Input: part model. Units: mm. Frame: model coordinates. Face numbers are marked on the shaded views. Coordinates: 2 decimals unless noted, no trailing zeros. Loops run counter-clockwise (first coordinate to the right, second up) from the corner with the lowest first, then second, coordinate; pieces in that order, holes last. Notation, with made-up numbers: (18.5, -21) - (62.5, -21) arc R24 ccw to (62.5, 3) - close; hole circle Ø11 at (79, 52.5). An arc over 180 degrees is marked (long way). Use a Markdown table: item, result. Add a question column.
1. Contact query for flat-ended pins moving along their axis: P1, Ø7.5, axis at x = 50.5, z = 7.5, coming from the -Y side; P2, Ø4, axis at x = -50.8, z = 6.35, coming from the +Y side; P3, Ø3, axis at x = 50.8, z = 6.35, coming from the -Y side (3 decimals); P4, Ø12, axis at x = -22.5, y = -18, coming from the -Z side. Output: stop coordinate, or through.
2. Section query B-B on z = 2. Return the cut outline in (x, y), then the cut area to 3 significant figures.
3. Section query C-C on x = 14.5. Return the cut outline in (y, z), then the cut area to 3 significant figures.
4. Ray query, L1, parallel to X at y = 37.25, z = 6.35; L2, parallel to Z at x = -50.8, y = 35.75. Return the intervals inside material, ascending. Write a range as [from, to].
5. Draft query along X for the marked faces 1, 2, 3 and 4. Return one class per face: released by +X, released by -X, zero draft, split by the parting line, or undercut.
6. Section query A-A on y = 34.5. Return the cut outline in (x, z).
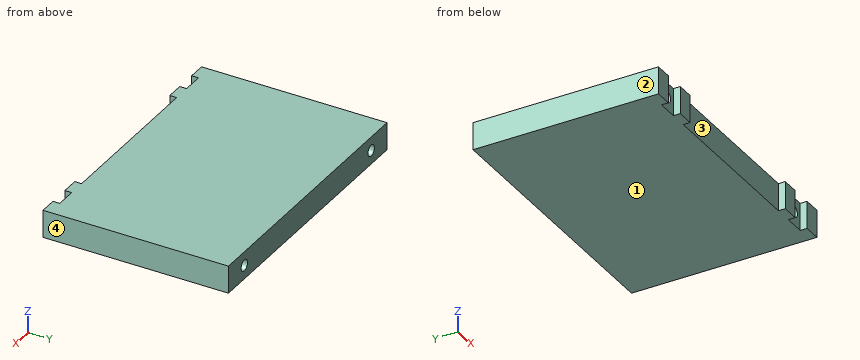
```python
from build123d import *

# Parameters (mm, degrees)
SKETCH1_W                   = 127
SKETCH1_H                   = 85.725
BOSS_EXTRUDE1_DEPTH         = 12.7
SKETCH2_W                   = 76.2
SKETCH2_H                   = 3.175
CUT_EXTRUDE1_DEPTH          = 78.657800035
SKETCH14_W                  = 9.525
SKETCH14_H                  = 3.175
CUT_EXTRUDE2_DEPTH          = 78.657800035
F_1_4_20_TAPPED_HOLE1_D     = 5.1054
F_1_4_20_TAPPED_HOLE1_DEPTH = 16.51
F_1_4_20_TAPPED_HOLE1_TIP   = 1.533816902
F_1_4_20_TAPPED_HOLE2_D     = 5.1054
F_1_4_20_TAPPED_HOLE2_DEPTH = 16.51
F_1_4_20_TAPPED_HOLE2_TIP   = 1.533816902


with BuildPart() as part:
    # Sketch1 → Boss-Extrude1 (new body)
    with BuildSketch(Plane.XY):
        Rectangle(SKETCH1_W, SKETCH1_H)
    extrude(amount=BOSS_EXTRUDE1_DEPTH)

    # Sketch2 → Cut-Extrude1 (cut, through all)
    with BuildSketch(Plane.XY.offset(12.7)):
        with Locations((0, -41.275)):
            Rectangle(SKETCH2_W, SKETCH2_H)
    extrude(amount=-CUT_EXTRUDE1_DEPTH, mode=Mode.SUBTRACT)

    # Sketch14 → Cut-Extrude2 (cut, through all)
    with BuildSketch(Plane.XY.offset(12.7)):
        with Locations((50.8, -41.275)):
            Rectangle(SKETCH14_W, SKETCH14_H)
        with Locations((-50.8, -41.275)):
            Rectangle(SKETCH14_W, SKETCH14_H)
    extrude(amount=-CUT_EXTRUDE2_DEPTH, mode=Mode.SUBTRACT)

    # 1/4-20 Tapped Hole1
    with Locations(Plane(origin=(-50.8, -39.6875, 6.35), x_dir=(-1, 0, 0), z_dir=(0, -1, 0))):
        with Locations((0, 0), (-101.6, 0)):
            Hole(F_1_4_20_TAPPED_HOLE1_D / 2, depth=F_1_4_20_TAPPED_HOLE1_DEPTH)
            with Locations((0, 0, -(F_1_4_20_TAPPED_HOLE1_DEPTH + F_1_4_20_TAPPED_HOLE1_TIP / 2))):  # 118° drill point
                Cone(0, F_1_4_20_TAPPED_HOLE1_D / 2, F_1_4_20_TAPPED_HOLE1_TIP, mode=Mode.SUBTRACT)

    # 1/4-20 Tapped Hole2
    with Locations(Plane(origin=(-50.8, 42.8625, 6.35), x_dir=(0, 0, 1), z_dir=(0, 1, 0))):
        with Locations((0, 0), (0, 101.6)):
            Hole(F_1_4_20_TAPPED_HOLE2_D / 2, depth=F_1_4_20_TAPPED_HOLE2_DEPTH)
            with Locations((0, 0, -(F_1_4_20_TAPPED_HOLE2_DEPTH + F_1_4_20_TAPPED_HOLE2_TIP / 2))):  # 118° drill point
                Cone(0, F_1_4_20_TAPPED_HOLE2_D / 2, F_1_4_20_TAPPED_HOLE2_TIP, mode=Mode.SUBTRACT)


solid = part.part
```
Resolved:
| question | item | result |
|---|---|---|
| 1 | P1 | y = -39.69 |
| 1 | P2 | y = 26.02 |
| 1 | P3 | y = -22.545 |
| 1 | P4 | z = 0 |
| 2 | outline | (-63.5, -42.86) - (-55.56, -42.86) - (-55.56, -39.69) - (-46.04, -39.69) - (-46.04, -42.86) - (-38.1, -42.86) - (-38.1, -39.69) - (38.1, -39.69) - (38.1, -42.86) - (46.04, -42.86) - (46.04, -39.69) - (55.56, -39.69) - (55.56, -42.86) - (63.5, -42.86) - (63.5, 42.86) - (-63.5, 42.86) - close |
| 2 | area | 10,600 mm² |
| 3 | outline | (-39.69, 0) - (42.86, 0) - (42.86, 12.7) - (-39.69, 12.7) - close |
| 3 | area | 1,050 mm² |
| 4 | L1 | [-63.5, -53.35], [-48.25, 48.25], [53.35, 63.5] |
| 4 | L2 | [0, 3.8], [8.9, 12.7] |
| 5 | face 1 | zero draft |
| 5 | face 2 | released by -X |
| 5 | face 3 | undercut |
| 5 | face 4 | released by +X |
| 6 | outline | (-63.5, 0) - (63.5, 0) - (63.5, 12.7) - (-63.5, 12.7) - close; hole circle Ø5.11 at (-50.8, 6.35); hole circle Ø5.11 at (50.8, 6.35) |
